Work out the finished part from the listing and answer in its coordinate system (mm). A direction names the side the tool comes from. Round coordinates to 2 decimals unless told otherwise and drop trailing zeros. Order: outer loops, then holes, each group sorted by start corner. A loop starts at its lowest first (then second) coordinate and runs counter-clockwise, first axis right, second up. Notation, with made-up numbers: M 24.5,84.25 L 79.5,84.25 A26 cw 79.5,106.25 Z; hole C 1.5,69 d10. An arc over 180 degrees is marked long. Return JSON: item names as keys, results as strings.
Autodesk Inventor part; units mm, degrees
ref_plane "YZ Plane" through (0, 0, 0) normal (1, 0, 0) x (0, 1, 0)
ref_plane "XZ Plane" through (0, 0, 0) normal (0, 1, 0) x (-1, 0, 0)
ref_plane "XY Plane" through (0, 0, 0) normal (0, 0, 1) x (1, 0, 0)
sketch "スケッチ2" plane through (0, 0, 0) normal (0, 1, 0) x (-1, 0, 0)
  line L0 (0, 0) -> (-77.8, 0)
  line L1 (-77.8, 0) -> (-77.8, -40)
  line L2 (-77.8, -40) -> (0, -40)
  line L3 (0, -40) -> (0, 0)
  dimension "d0" = 77.8
  dimension "d1" = 40
extrude "押し出し1" add sketch "スケッチ2" along normal blind 5
sketch "スケッチ4" plane through (0, 0, -40) normal (-1, 0, 0) x (0, 0, 1)
  line L0 (0, 0) -> (0, 5) construction
  line L1 (0, 2.5) -> (40, 2.5) construction
  line L2 (40, 0) -> (40, 5) construction
  point P0 (4, 2.5)
  point P1 (36, 2.5)
  dimension "d4" = 4
  dimension "d5" = 4
hole "穴1" at (0, 2.5, -36) at (0, 2.5, -4) direction (1, 0, 0) diameter 2.459 depth 12
sketch "スケッチ5" plane through (77.8, 0, 0) normal (1, 0, 0) x (0, 0, -1)
  line L0 (0, 0) -> (0, 5) construction
  line L1 (0, 2.5) -> (39.9198, 2.5) construction
  circle A0 centre (4, 2.5) radius 1.2295 construction
  circle A1 centre (36, 2.5) radius 1.2295
hole "穴2" at (77.8, 2.5, -4) at (77.8, 2.5, -36) direction (-1, 0, 0) diameter 2.459 depth 13
sketch "スケッチ6" plane through (0, 5, 0) normal (0, 1, 0) x (1, 0, 0)
  line L0 (77.8, 0) -> (77.8, 40) construction
  line L1 (0, 40) -> (0, 0) construction
  line L2 (0, 0) -> (77.8, 0) construction
  point P0 (57.3, 12.5)
  dimension "d20" = 20.5
  dimension "d21" = 12.5
hole "穴3" at (57.3, 5, -12.5) direction (0, -1, 0) diameter 8.5 end through all
sketch "スケッチ7" plane through (0, 5, 0) normal (0, 1, 0) x (1, 0, 0)
  circle A0 centre (57.3, 12.5) radius 4.25 construction
  circle A1 centre (57.3, 12.5) radius 7 construction
  point P0 (0, 0)
  point P1 (64.3, 12.5)
  point P2 (57.3, 19.5)
  point P3 (57.3, 5.5)
  dimension "d29" = 14
hole "穴4" at (64.3, 5, -12.5) at (57.3, 5, -19.5) at (57.3, 5, -5.5) direction (0, -1, 0) diameter 2.459 end through all
sketch "スケッチ9" plane through (0, 5, 0) normal (0, 1, 0) x (1, 0, 0)
  circle A0 centre (57.3, 12.5) radius 4.25 construction
  line L0 (57.3, 12.5) -> (44.1485, 12.5) construction
  line L1 (50.05, 13.2) -> (53.05, 13.2)
  line L2 (53.05, 13.2) -> (53.05, 11.8)
  line L3 (53.05, 11.8) -> (50.05, 11.8)
  line L4 (50.05, 11.8) -> (50.05, 13.2)
  line L5 (50.05, 13.2) -> (53.05, 11.8) construction
  line L6 (53.05, 13.2) -> (50.05, 11.8) construction
  line L7 (53.05, 11.8) -> (53.108, 11.8)
  line L8 (53.05, 13.2) -> (53.108, 13.2)
  point P0 (0, 0)
  point P1 (51.55, 12.5)
  dimension "d41" = 3
  dimension "d42" = 1.4
  dimension "d43" = 0
properties part number "shoulder1_verticval_left_cover" material "アルミニウム 5052"
Item 1: Find section A-A (z = -16). Determine the outline of the cut face in (x, y), plus the area to 3 significant figures.
Output:
{"outline": "M 0,0 L 54.89,0 L 54.89,5 L 0,5 Z; M 59.71,0 L 77.8,0 L 77.8,5 L 59.71,5 Z", "area": "365 mm^2"}
Item 2: Consider line 1 along Z through (x, y) = (57.3, 2.4); line 2 along Z through (x, y) = (74, 2.5); line 3 along X through (y, z) = (2.35, -19.5). Determine where each line is inside the solid, lowest interval first. Write a range as [from, to].
Output:
{"line 1": "z = [-40, -20.73], [-18.27, -16.75], [-8.25, -6.73], [-4.27, 0]", "line 2": "z = [-40, -37.23], [-34.77, -5.23], [-2.77, 0]", "line 3": "x = [0, 56.07], [58.53, 77.8]"}
Item 3: Each of these flat-tipped pins is pushed along its axis until it touches: pin 1 (1.2 mm diameter, centred on y = 2.5, z = -36.5, fed in from +X); pin 2 (2 mm diameter, centred on y = 2.5, z = -4, fed in from -X). Where does it stop, or does it pass through?
Output:
{"pin 1": "stops at x = 64.8", "pin 2": "stops at x = 12"}
Item 4: Find section B-B (x = 57.3). Determine the outline of the cut face in (y, z), plus the area to 3 significant figures.
Output:
{"outline": "M 0,-40 L 5,-40 L 5,-20.73 L 0,-20.73 Z; M 0,-18.27 L 5,-18.27 L 5,-16.75 L 0,-16.75 Z; M 0,-8.25 L 5,-8.25 L 5,-6.73 L 0,-6.73 Z; M 0,-4.27 L 5,-4.27 L 5,0 L 0,0 Z", "area": "133 mm^2"}
Item 5: The mould has two halves that part along Z. Classify faces 1 (the flat face through (39, 2, -40)), 2 (the flat face through (39, 0, -20)), 3 (the cylindrical face through (6.084, 2.131, -34.827)), 4 (the flat face through (38, 2, 0)): pulls with the +Z half, pulls with the -Z half, needs draft (parallel to the pull), parting line crosses it, or undercut.
Output:
{"face 1": "pulls with the -Z half", "face 2": "needs draft", "face 3": "undercut", "face 4": "pulls with the +Z half"}
Item 6: Find section C-C (z = -36). Determine the outline of the cut face in (x, y).
Output:
{"outline": "M 0,0 L 77.8,0 L 77.8,1.27 L 64.8,1.27 L 64.8,3.73 L 77.8,3.73 L 77.8,5 L 0,5 L 0,3.73 L 12,3.73 L 12,1.27 L 0,1.27 Z"}
Item 7: Which of the six approach directions +Z, -Z, +X, -X, +Y, -Y give full straight-line access (tool end or side, diameter ignored) to faces 5 (the flat face through (64.8, 2, -4)), 6 (the flat face through (77.8, 2, -20)), 7 (the cylindrical face through (6.08, 2.45, -5.23))?
Output:
{"face 5": "+X", "face 6": "+Z, -Z, +X, +Y, -Y", "face 7": "-X"}
